from build123d import *

# Parameters (mm, degrees)
RESSALTO_EXTRUS_O2_DEPTH                   = 10
BROCA_DE_ROSQUEAR_PARA_TARRAXA_DE_M4X0_7_D = 3.3
BROCA_DE_ROSQUEAR_PARA_TARRAXA_DE_M4_2_D   = 3.3


with BuildPart() as part:
    # Esboço1 → Ressalto-extrusão2 (new body)
    with BuildSketch(Plane.XY):
        Polygon((0, 0), (15, 0), (15, 2), (2, 2), (2, 15), (0, 15), align=None)
    extrude(amount=RESSALTO_EXTRUS_O2_DEPTH)

    # Broca de rosquear para tarraxa de M4x0.7 (through all)
    with Locations(Plane(origin=(2, 10, 5), x_dir=(0, 0, 1), z_dir=(1, 0, 0))):
        with Locations((0, 0)):
            Hole(BROCA_DE_ROSQUEAR_PARA_TARRAXA_DE_M4X0_7_D / 2)

    # Broca de rosquear para tarraxa de M4 2 (through all)
    with Locations(Plane(origin=(10, 0, 5), x_dir=(0, 0, -1), z_dir=(0, -1, 0))):
        with Locations((0, 0)):
            Hole(BROCA_DE_ROSQUEAR_PARA_TARRAXA_DE_M4_2_D / 2)


solid = part.part
CAD build for the part. Positions are in the model's coordinates, mm. A direction names the side the tool comes from. Round coordinates to 2 decimals unless told otherwise and drop trailing zeros. Order: outer loops, then holes, each group sorted by start corner. A loop starts at its lowest first (then second) coordinate and runs counter-clockwise, first axis right, second up. Notation, with made-up numbers: (7.5, -9.5) - (19.5, -9.5) arc R31 ccw to (19.5, 17.5) - close; hole circle Ø8 at (-21, 88.5). An arc over 180 degrees is marked (long way). Return JSON: item names as keys, results as strings.
(1) Pull direction Z, two halves, no side cores. Call faces 3 (the face through (1, 5, 10)), 4 (the face through (9, 1.01, 3.69)), 5 (the face through (0, 8, 5)): +Z half, -Z half, draft (parallel to the pull), parting line (faces both ways), or undercut.
Answer key:
{"face 3": "+Z half", "face 4": "undercut", "face 5": "draft"}
(2) Cut at A-A (x = 10). Give the cut face in (y, z).
Answer key:
{"outline": "(0, 0) - (2, 0) - (2, 3.35) - (0, 3.35) - close; (0, 6.65) - (2, 6.65) - (2, 10) - (0, 10) - close"}
(3) Pin check, flat tips, straight feed: pin 1 Ø4 at (x, z) = (5.5, 6.5) entering from +Y; pin 2 Ø3 at (x, z) = (10, 5) entering from +Y; pin 3 Ø2 at (y, z) = (12, 6.5) entering from +X. Stop position of each tip, or through.
Answer key:
{"pin 1": "stops at y = 2", "pin 2": "passes through", "pin 3": "stops at x = 2"}
(4) Cut at D-D (z = 2.75). Give the cut face in (x, y), then the cut area to 3 significant figures.
Answer key:
{"outline": "(0, 0) - (15, 0) - (15, 2) - (2, 2) - (2, 15) - (0, 15) - close", "area": "56.0 mm^2"}
(5) Wall check: probe 1 along Z at (x, y) = (0.95, 10); probe 2 along X at (y, z) = (0.7, 5); probe 3 along Y at (x, z) = (7.5, 4.5). Give the ranges that are in metal, low to high. Write a range as from..to.
Answer key:
{"probe 1": "z = 0..3.35, 6.65..10", "probe 2": "x = 0..8.35, 11.65..15", "probe 3": "y = 0..2"}
(6) Cut at B-B (z = 5). Give the cut face in (x, y).
Answer key:
{"outline": "(0, 0) - (8.35, 0) - (8.35, 2) - (2, 2) - (2, 8.35) - (0, 8.35) - close; (0, 11.65) - (2, 11.65) - (2, 15) - (0, 15) - close; (11.65, 0) - (15, 0) - (15, 2) - (11.65, 2) - close"}
(7) Tool access for faces 1 (the face through (15, 1, 5)), 2 (the face through (8.6, 2, 3.8)): list every direction of +Z, -Z, +X, -X, +Y, -Y with a clear straight run to the whole face (end or side of a thin tool).
Answer key:
{"face 1": "+Z, -Z, +X, +Y, -Y", "face 2": "+Z, -Z, +X, +Y"}
